The model under review builds one solid part; all positions refer to its coordinate system, in mm. Face numbers are marked on the shaded views. A direction names the side the tool comes from. Coordinates: 2 decimals unless noted, no trailing zeros. Write each loop counter-clockwise with the first axis right and the second up, starting at its lowest first coordinate (ties: lowest second). Pieces come first, ordered by that corner, then holes.
```python
from build123d import *

# Parameters (mm, degrees)
SKETCH1_R               = 9.55
BOSS_EXTRUDE1_DEPTH     = 2.6
SKETCH2_R               = 4.5
BOSS_EXTRUDE2_DEPTH     = 1.29
CUT_EXTRUDE1_DEPTH      = 15.054789219
CUT_EXTRUDE1_DEPTH_BACK = 3.39
SKETCH3_R               = 2.72
SKETCH4_R               = 1.4
CUT_EXTRUDE2_DEPTH      = 14.753726768


with BuildPart() as part:
    # Sketch1 → Boss-Extrude1 (new body)
    with BuildSketch(Plane(origin=(0, 0, 0), x_dir=(1, 0, 0), z_dir=(0, 1, 0))):
        with Locations(Location((0, 0, 0), (0, 0, 270))):
            Circle(SKETCH1_R)
    extrude(amount=BOSS_EXTRUDE1_DEPTH)

    # Sketch2 → Boss-Extrude2 (add)
    with BuildSketch(Plane(origin=(0, 2.6, 0), x_dir=(1, 0, 0), z_dir=(0, 1, 0))):
        with Locations(Location((0, 0, 0), (0, 0, 270))):
            Circle(SKETCH2_R)
    extrude(amount=BOSS_EXTRUDE2_DEPTH)

    # Sketch3 → Cut-Extrude1 (cut, two sides: drawn at the far end of the back side and taken through both)
    with BuildSketch(Plane(origin=(0, 3.89, 0), x_dir=(1, 0, 0), z_dir=(0, 1, 0)).offset(-CUT_EXTRUDE1_DEPTH_BACK)):
        with Locations(Location((0, 0, 0), (0, 0, 270))):
            Circle(SKETCH3_R)
    extrude(amount=CUT_EXTRUDE1_DEPTH + CUT_EXTRUDE1_DEPTH_BACK, mode=Mode.SUBTRACT)

    # Sketch4 → Cut-Extrude2 (cut, through all)
    with BuildSketch(Plane(origin=(0, 2.6, 0), x_dir=(1, 0, 0), z_dir=(0, 1, 0))):
        with Locations(Location((0, 6.95, 0), (0, 0, 270))):
            Circle(SKETCH4_R)
        with Locations(Location((6.95, 0, 0), (0, 0, 270))):
            Circle(SKETCH4_R)
        with Locations(Location((0, -6.95, 0), (0, 0, 270))):
            Circle(SKETCH4_R)
        with Locations(Location((-6.95, 0, 0), (0, 0, 270))):
            Circle(SKETCH4_R)
    extrude(amount=-CUT_EXTRUDE2_DEPTH, mode=Mode.SUBTRACT)


solid = part.part
```
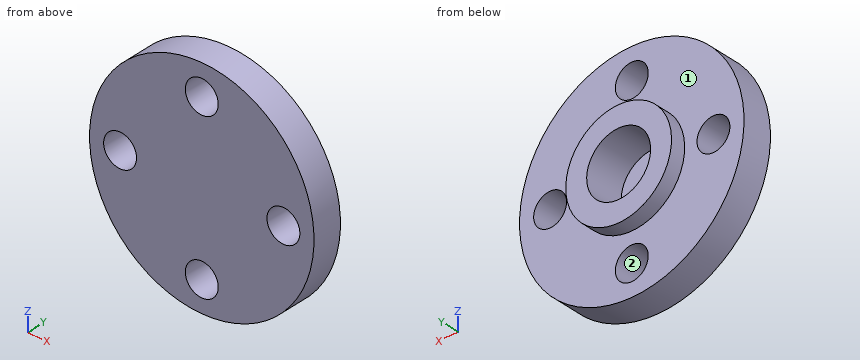
Item 1: To check wall thickness, follow line 1 along X through (y, z) = (0.7, 0); line 2 along X through (y, z) = (0.6, 0.75); line 3 along Z through (x, y) = (-1.25, 0.2). State the ranges of each line that lie inside material, in increasing order.
Solved:
line 1: x = -9.55 to -8.35, -5.55 to -2.72, 2.72 to 5.55, 8.35 to 9.55
line 2: x = -9.52 to -8.13, -5.77 to -2.61, 2.61 to 5.77, 8.13 to 9.52
line 3: z = -9.47 to -7.58, -6.32 to 6.32, 7.58 to 9.47
Item 2: Take a section at D-D, the plane x = 6.95. Write out the cut boundary in (y, z), plus the area to 3 significant figures.
Solved:
outline: (0, -6.55) - (2.6, -6.55) - (2.6, -1.4) - (0, -1.4) - close; (0, 1.4) - (2.6, 1.4) - (2.6, 6.55) - (0, 6.55) - close
area: 26.8 mm2
Item 3: Take a section at B-B, the plane x = 0. Write out the cut boundary in (y, z).
Solved:
outline: (0, -9.55) - (2.6, -9.55) - (2.6, -8.35) - (0, -8.35) - close; (0, -5.55) - (2.6, -5.55) - (2.6, -4.5) - (3.89, -4.5) - (3.89, -2.72) - (0.5, -2.72) - (0.5, 2.72) - (3.89, 2.72) - (3.89, 4.5) - (2.6, 4.5) - (2.6, 5.55) - (0, 5.55) - close; (0, 8.35) - (2.6, 8.35) - (2.6, 9.55) - (0, 9.55) - close
Item 4: For pin 1 (4.5 mm diameter, centred on x = 0, z = -6.95, fed in from +Y); pin 2 (2.5 mm diameter, centred on x = -6.95, z = 0, fed in from +Y); pin 3 (2 mm diameter, centred on x = 4.5, y = 2.5, fed in from +Z), all flat-tipped, find the tip position at first contact; note any pin that passes through.
Solved:
pin 1: stops at y = 2.6
pin 2: passes through
pin 3: stops at z = 8.89
Item 5: Take a section at C-C, the plane y = 1.1. Write out the cut boundary in (x, z).
Solved:
outline: circle Ø19.1 at (0, 0); hole circle Ø2.8 at (-6.95, 0); hole circle Ø5.44 at (0, 0); hole circle Ø2.8 at (0, -6.95); hole circle Ø2.8 at (0, 6.95); hole circle Ø2.8 at (6.95, 0)
Item 6: Machinability: for the marked faces 1 and 2, which of the approach directions +Z, -Z, +X, -X, +Y, -Y give a long, thin tool a straight path to every point of the face, cutting with its end or side? Answer none if there is none.
Solved:
face 1: +Y
face 2: +Y, -Y
Item 7: Take a section at A-A, the plane z = 0. Write out the cut boundary in (x, y), plus the area to 3 significant figures.
Solved:
outline: (-9.55, 0) - (-8.35, 0) - (-8.35, 2.6) - (-9.55, 2.6) - close; (-5.55, 0) - (5.55, 0) - (5.55, 2.6) - (4.5, 2.6) - (4.5, 3.89) - (2.72, 3.89) - (2.72, 0.5) - (-2.72, 0.5) - (-2.72, 3.89) - (-4.5, 3.89) - (-4.5, 2.6) - (-5.55, 2.6) - close; (8.35, 0) - (9.55, 0) - (9.55, 2.6) - (8.35, 2.6) - close
area: 28.3 mm2
